The model under review builds one solid part; all positions refer to its coordinate system, in mm. A direction names the side the tool comes from. Coordinates: 2 decimals unless noted, no trailing zeros. Write each loop counter-clockwise with the first axis right and the second up, starting at its lowest first coordinate (ties: lowest second). Pieces come first, ordered by that corner, then holes. Notation, with made-up numbers: (50.25, 70.5) - (62.25, 70.5) arc R26 ccw to (62.25, 102.5) - close; hole circle Ø4 at (31, -10.5). An arc over 180 degrees is marked (long way). Put each result on its own line as item: value. Start each with the question number.
Item 1: Consider section A-A on z = 146. Give the boundary of the cut face in (x, y).
Item 2: Consider section D-D on z = 13.5. Give the boundary of the cut face in (x, y).
Item 3: Consider section C-C on x = -114. Give the boundary of the cut face in (y, z).
Item 4: Consider section B-B on y = -593. Give the boundary of the cut face in (x, z), then the cut area to 3 significant figures.
Item 5: For pin 1 (12 mm diameter, centred on x = 185.5, z = 148, fed in from +Y); pin 2 (5 mm diameter, centred on x = -70.5, y = 231.5, fed in from +Z); pin 3 (5 mm diameter, centred on y = -220, z = 107, fed in from -X), all flat-tipped, find the tip position at first contact; note any pin that passes through.
Item 6: Mouldability with a two-part tool opening along X and no side actions: class faces 5 (the face through (-401.205, -193, 111)), 6 (the face through (-321.92, 344.62, 14.79)), 7 (the face through (188.86, -392.62, 115.92)) as pulls with the +X half, pulls with the -X half, needs draft (parallel to the pull), parting line crosses it, or undercut.
Item 7: Machinability: for faces 1 (the face through (-196.205, 430, 111)), 2 (the face through (255.35, 106.32, 115.92)), 3 (the face through (238.795, -188, 116)), 4 (the face through (182.79, -382.46, 110.85)), which of the approach directions +Z, -Z, +X, -X, +Y, -Y give a long, thin tool a straight path to every point of the face, cutting with its end or side? Answer none if there is none.
Item 8: To check wall thickness, follow L1, parallel to Z at x = -99, y = -681; L2, parallel to Z at x = 48.5, y = -131.5; L3, parallel to Y at x = -135, z = 27. State the ranges of each line that lie inside material, in increasing order. Write a range as [from, to].
```python
from build123d import *
from build123d.topology import SkipClean

# Parameters (mm, degrees)
PIASTRONEEXTR_DEPTH   = 30
LAMONE_DEPTH          = 40
CARTEREXT1_START      = 30
CARTEREXT1_DEPTH      = 10
CARTEREXT2_START      = 40
CARTEREXT2_DEPTH      = 154
IRRIGIDCIRC1_START    = 30
IRRIGIDCIRC1_DEPTH    = 10
IRRIGIDCIRC2_START    = 40
IRRIGIDCIRC2_DEPTH    = 154
IRRIGIDESTERNO1_START = 30
IRRIGIDESTERNO1_DEPTH = 10
IRRIGIDESTERNO2_START = 40
IRRIGIDESTERNO2_DEPTH = 154
RINFORZOSUP1_START    = 30
SKETCH12_W            = 110
SKETCH12_H            = 85
RINFORZOSUP1_DEPTH    = 20
BOSS_EXTRUDE1_START   = 50
SKETCH12_4_W          = 110
SKETCH12_4_H          = 45
BOSS_EXTRUDE1_DEPTH   = 144


with BuildPart() as part:
    # Piastrone → PiastroneExtr (new body)
    with BuildSketch(Plane.XY):
        with BuildLine():
            Line((-86.205427068, 491.905049747), (23.794572932, 491.905049747))
            Line((23.794572932, 491.905049747), (278.794572932, 193.153386451))
            Line((278.794572932, 193.153386451), (278.794572932, -303.297278914))
            Line((278.794572932, -303.297278914), (23.794572932, -808.094950253))
            Line((23.794572932, -808.094950253), (-86.205427068, -808.094950253))
            Line((-86.205427068, -808.094950253), (-86.205427068, -620.594950253))
            ThreePointArc((-86.205427068, -620.594950253), (-33.705427068, -568.094950253), (-86.205427068, -515.594950253))
            Line((-86.205427068, -515.594950253), (-86.205427068, 21.905049747))
            ThreePointArc((-86.205427068, 21.905049747), (-21.205427068, 86.905049747), (-86.205427068, 151.905049747))
            Line((-86.205427068, 151.905049747), (-86.205427068, 491.905049747))
        make_face()
    extrude(amount=PIASTRONEEXTR_DEPTH)


with BuildPart() as body_2:
    # Sketch14 → Lamone (new body)
    with BuildSketch(Plane(origin=(0, 0, 0), x_dir=(-1, 0, 0), z_dir=(0, 0, -1))):
        with BuildLine():
            Line((-23.794572932, 491.905049747), (86.205427068, 491.905049747))
            Line((86.205427068, 491.905049747), (86.205427068, 151.905049747))
            ThreePointArc((86.205427068, 151.905049747), (21.205427068, 86.905049747), (86.205427068, 21.905049747))
            Line((86.205427068, 21.905049747), (86.205427068, -515.594950253))
            ThreePointArc((86.205427068, -515.594950253), (33.705427068, -568.094950253), (86.205427068, -620.594950253))
            Line((86.205427068, -620.594950253), (86.205427068, -808.094950253))
            Line((86.205427068, -808.094950253), (-23.794572932, -808.094950253))
            Line((-23.794572932, -808.094950253), (-23.794572932, 491.905049747))
        make_face()
    extrude(amount=LAMONE_DEPTH)


with BuildPart() as body_3:
    # Carter → CarterExt1 (new body)
    with BuildSketch(Plane.XY.offset(CARTEREXT1_START)):
        with BuildLine():
            ThreePointArc((248.758008424, 81.95561707), (255.585083182, 106.603061749), (278.794572932, 117.346667498))
            Line((278.794572932, 117.346667498), (278.794572932, 86.905049747))
            ThreePointArc((278.794572932, 86.905049747), (171.888548065, -171.188925386), (-86.205427068, -278.094950253))
            Line((-86.205427068, -278.094950253), (-86.205427068, -248.094950253))
            ThreePointArc((-86.205427068, -248.094950253), (148.918944333, -151.719194564), (248.758008424, 81.95561707))
        make_face()
        with BuildLine():
            ThreePointArc((-86.205427068, -248.094950253), (148.918944333, -151.719194564), (248.758008424, 81.95561707))
            ThreePointArc((248.758008424, 81.95561707), (255.585083182, 106.603061749), (278.794572932, 117.346667498))
            Line((278.794572932, 117.346667498), (278.794572932, 127.247815787))
            ThreePointArc((278.794572932, 127.247815787), (248.567893296, 113.623706335), (238.756848588, 81.953342871))
            ThreePointArc((238.756848588, 81.953342871), (141.846864376, -144.648728817), (-86.205427068, -238.094950253))
            Line((-86.205427068, -238.094950253), (-86.205427068, -248.094950253))
        make_face()
    extrude(amount=CARTEREXT1_DEPTH)

    # Carter<4> → CarterExt2 (add)
    with BuildSketch(Plane.XY.offset(CARTEREXT2_START)):
        with BuildLine():
            ThreePointArc((-86.205427068, -248.094950253), (148.918944333, -151.719194564), (248.758008424, 81.95561707))
            ThreePointArc((248.758008424, 81.95561707), (255.585083182, 106.603061749), (278.794572932, 117.346667498))
            Line((278.794572932, 117.346667498), (278.794572932, 127.247815787))
            ThreePointArc((278.794572932, 127.247815787), (248.567893296, 113.623706335), (238.756848588, 81.953342871))
            ThreePointArc((238.756848588, 81.953342871), (141.846864376, -144.648728817), (-86.205427068, -238.094950253))
            Line((-86.205427068, -238.094950253), (-86.205427068, -248.094950253))
        make_face()
    extrude(amount=CARTEREXT2_DEPTH)


with BuildPart() as body_4:
    # IrrigidCirc → IrrigidCirc1 (new body)
    with BuildSketch(Plane.XY.offset(IRRIGIDCIRC1_START)):
        with BuildLine():
            ThreePointArc((-86.205427068, -338.094950253), (77.301662182, -406.337626569), (143.781261282, -570.569456643))
            Line((143.781261282, -570.569456643), (115.484539714, -626.585610189))
            ThreePointArc((115.484539714, -626.585610189), (81.697876334, -441.966124417), (-86.205427068, -358.094950253))
            Line((-86.205427068, -358.094950253), (-86.205427068, -338.094950253))
        make_face()
        with BuildLine():
            ThreePointArc((-86.205427068, -328.094950253), (77.651833725, -392.735895495), (153.243359331, -551.838299541))
            Line((153.243359331, -551.838299541), (143.781261282, -570.569456643))
            ThreePointArc((143.781261282, -570.569456643), (77.301662182, -406.337626569), (-86.205427068, -338.094950253))
            Line((-86.205427068, -338.094950253), (-86.205427068, -328.094950253))
        make_face()
    extrude(amount=IRRIGIDCIRC1_DEPTH)

    # IrrigidCirc<7> → IrrigidCirc2 (add)
    with BuildSketch(Plane.XY.offset(IRRIGIDCIRC2_START)):
        with BuildLine():
            ThreePointArc((-86.205427068, -328.094950253), (77.651833725, -392.735895495), (153.243359331, -551.838299541))
            Line((153.243359331, -551.838299541), (143.781261282, -570.569456643))
            ThreePointArc((143.781261282, -570.569456643), (77.301662182, -406.337626569), (-86.205427068, -338.094950253))
            Line((-86.205427068, -338.094950253), (-86.205427068, -328.094950253))
        make_face()
    extrude(amount=IRRIGIDCIRC2_DEPTH)


with BuildPart() as body_5:
    # Sketch9 → IrrigidEsterno1 (new body)
    with BuildSketch(Plane.XY.offset(IRRIGIDESTERNO1_START)):
        with BuildLine():
            Line((238.794572932, -293.767656293), (278.794572932, -303.297278914))
            Line((278.794572932, -303.297278914), (278.794572932, 86.905049747))
            ThreePointArc((278.794572932, 86.905049747), (268.653699911, 1.465012294), (238.794572932, -79.227427511))
            Line((238.794572932, -79.227427511), (238.794572932, -293.767656293))
        make_face()
        with BuildLine():
            Line((153.243359331, -551.838299541), (278.794572932, -303.297278914))
            Line((278.794572932, -303.297278914), (238.794572932, -293.767656293))
            Line((238.794572932, -293.767656293), (140.299029593, -488.749306939))
            ThreePointArc((140.299029593, -488.749306939), (148.897021721, -519.857635093), (153.243359331, -551.838299541))
        make_face()
        with BuildLine():
            Line((140.299029593, -488.749306939), (238.794572932, -293.767656293))
            Line((238.794572932, -293.767656293), (228.794572932, -291.385250638))
            Line((228.794572932, -291.385250638), (135.473141453, -476.124236116))
            ThreePointArc((135.473141453, -476.124236116), (137.974978228, -482.402792609), (140.299029593, -488.749306939))
        make_face()
        with BuildLine():
            Line((228.794572932, -291.385250638), (238.794572932, -293.767656293))
            Line((238.794572932, -293.767656293), (238.794572932, -79.227427511))
            ThreePointArc((238.794572932, -79.227427511), (233.924768948, -88.42794087), (228.794572932, -97.485839398))
            Line((228.794572932, -97.485839398), (228.794572932, -291.385250638))
        make_face()
    extrude(amount=IRRIGIDESTERNO1_DEPTH)

    # Sketch9<3> → IrrigidEsterno2 (add)
    with BuildSketch(Plane.XY.offset(IRRIGIDESTERNO2_START)):
        with BuildLine():
            Line((228.794572932, -291.385250638), (238.794572932, -293.767656293))
            Line((238.794572932, -293.767656293), (238.794572932, -79.227427511))
            ThreePointArc((238.794572932, -79.227427511), (233.924768948, -88.42794087), (228.794572932, -97.485839398))
            Line((228.794572932, -97.485839398), (228.794572932, -291.385250638))
        make_face()
        with BuildLine():
            Line((140.299029593, -488.749306939), (238.794572932, -293.767656293))
            Line((238.794572932, -293.767656293), (228.794572932, -291.385250638))
            Line((228.794572932, -291.385250638), (135.473141453, -476.124236116))
            ThreePointArc((135.473141453, -476.124236116), (137.974978228, -482.402792609), (140.299029593, -488.749306939))
        make_face()
    extrude(amount=IRRIGIDESTERNO2_DEPTH)


with BuildPart() as body_6:
    # Sketch12 → RinforzoSup1 (new body)
    with BuildSketch(Plane.XY.offset(RINFORZOSUP1_START)):
        with Locations((-31.205427068, 449.405049747)):
            Rectangle(SKETCH12_W, SKETCH12_H)
    extrude(amount=RINFORZOSUP1_DEPTH)

    # Sketch12<4> → Boss-Extrude1 (add)
    with BuildSketch(Plane.XY.offset(BOSS_EXTRUDE1_START)):
        with Locations((-31.205427068, 429.405049747)):
            Rectangle(SKETCH12_4_W, SKETCH12_4_H)
    extrude(amount=BOSS_EXTRUDE1_DEPTH)


with BuildPart() as body_2_1:
    add(body_2.part)

    # Combine11: union part, body 6, body 3, body 5, body 4
    add(part.part)
    add(body_6.part)
    add(body_3.part)
    add(body_5.part)
    add(body_4.part)

    # Mirror3: body 2 across plane


with BuildPart() as body_2_2:
    with SkipClean():  # the faces are left unmerged after this step: merging them gives an invalid solid
        add(body_2_1.part)
        add(body_2_1.part.mirror(Plane(origin=(-86.205427068, 491.905049747, -40), x_dir=(0, 0, 1), z_dir=(1, 0, 0))))


solid = body_2_2.part
```
Report:
1. outline: (-451.21, 117.35) arc R30.44 cw to (-421.17, 81.96) arc R335 ccw to (248.76, 81.96) arc R30.44 cw to (278.79, 117.35) - (278.79, 127.25) arc R40.34 ccw to (238.76, 81.95) arc R325 cw to (-411.17, 81.95) arc R40.34 ccw to (-451.21, 127.25) - close; (-411.21, -293.77) - (-312.71, -488.75) arc R240 ccw to (-325.65, -551.84) - (-316.19, -570.57) arc R230 cw (long way) to (143.78, -570.57) - (153.24, -551.84) arc R240 ccw to (140.3, -488.75) - (238.79, -293.77) - (238.79, -79.23) arc R365 cw to (228.79, -97.49) - (228.79, -291.39) - (135.47, -476.12) arc R240 ccw to (-307.88, -476.12) - (-401.21, -291.39) - (-401.21, -97.49) arc R365 cw to (-411.21, -79.23) - close; (-196.21, 406.91) - (23.79, 406.91) - (23.79, 451.91) - (-196.21, 451.91) - close
2. outline: (-451.21, -303.3) - (-196.21, -808.09) - (23.79, -808.09) - (278.79, -303.3) - (278.79, 193.15) - (23.79, 491.91) - (-196.21, 491.91) - (-451.21, 193.15) - close; hole circle Ø130 at (-86.21, 86.91); hole circle Ø105 at (-86.21, -568.09)
3. outline: (-808.09, -40) - (-612.63, -40) - (-612.63, 30) - (-808.09, 30) - close; (-523.56, -40) - (28.15, -40) - (28.15, 30) - (-236.9, 30) - (-236.9, 194) - (-246.94, 194) - (-246.94, 40) - (-277.04, 40) - (-277.04, 30) - (-329.71, 30) - (-329.71, 194) - (-339.78, 194) - (-339.78, 40) - (-359.94, 40) - (-359.94, 30) - (-523.56, 30) - close; (145.66, -40) - (491.91, -40) - (491.91, 50) - (451.91, 50) - (451.91, 194) - (406.91, 194) - (406.91, 30) - (145.66, 30) - close
4. outline: (-304.86, 0) - (-196.21, 0) - (-196.21, -40) - (-132.42, -40) - (-132.42, 30) - (-294.72, 30) - (-294.72, 40) - (-304.86, 40) - close; (-39.99, -40) - (23.79, -40) - (23.79, 0) - (132.45, 0) - (132.45, 40) - (122.31, 40) - (122.31, 30) - (-39.99, 30) - close
4. area: 15,700 mm²
5. pin 1: y = -81.93
5. pin 2: z = 30
5. pin 3: x = -411.21
6. face 5: undercut
6. face 6: pulls with the -X half
6. face 7: pulls with the +X half
7. face 1: +Z, -X, +Y
7. face 2: +Z, +X
7. face 3: +Z, +X, -Y
7. face 4: +Z
8. L1: [-40, 30]
8. L2: [0, 30]
8. L3: [-808.09, -587.47], [-548.72, 43.96], [129.85, 491.91]
